```python
from build123d import *

# Parameters (mm, degrees)
F0_R     = 142.5
F1_DEPTH = 100
F2_R     = 100
F3_DEPTH = 75
F4_R     = 50
F5_DEPTH = 50


with BuildPart() as f1:
    # F0 (on Front) → F1 (new body)
    with BuildSketch(Plane.XZ):
        Circle(F0_R)
    extrude(amount=F1_DEPTH)

    # F2 (on face) → F3 (cut)
    with BuildSketch(Plane.XZ.offset(100)):
        Circle(F2_R)
    extrude(amount=-F3_DEPTH, mode=Mode.SUBTRACT)

    # F4 (on face) → F5 (join)
    with BuildSketch(Plane.XZ.offset(25)):
        Circle(F4_R)
    extrude(amount=F5_DEPTH)


solid = f1.part
```
For this review, take the finished solid that the model builds, in its own axes (mm). A direction names the side the tool comes from. Give positions to 0.01 mm unless a question says otherwise; leave off trailing zeros. Write each loop counter-clockwise with the first axis right and the second up, starting at its lowest first coordinate (ties: lowest second). Pieces come first, ordered by that corner, then holes. Notation, with made-up numbers: M 10.25,-13 L 53.25,-13 A26 ccw 53.25,15 Z; hole C 70,9.5 d3. An arc over 180 degrees is marked long. Answer as a JSON object with one key per item and string values. Group by question number.
Item 1: Consider section D-D on y = -86. Write out the cut boundary in (x, z), plus the area to 3 significant figures.
Item 2: For pin 1 Ø1.5 at (y, z) = (-85, -19.5) entering from +X; pin 2 Ø12 at (y, z) = (-79, -18) entering from +X; pin 3 Ø1 at (y, z) = (-19, -59.5) entering from +X, all flat-tipped, find the tip position at first contact; note any pin that passes through.
Item 3: For probe 1 along Z at (x, y) = (0, -73.5); probe 2 along Y at (x, z) = (67, 68); probe 3 along X at (y, z) = (-29.5, -51.5), list the stretches that pass through material, from the lowest coordinate up. Write a range as [from, to].
Item 4: Consider section C-C on z = 0. Write out the cut boundary in (x, y), plus the area to 3 significant figures.
Item 5: Consider section A-A on y = -70.5. Write out the cut boundary in (x, z), plus the area to 3 significant figures.
Item 6: Tool access review of faces 1 (the flat face through (-2, 0, 2)), 2 (the cylindrical face through (95.38, -63.02, 30.04)): name each direction out of +Z, -Z, +X, -X, +Y, -Y from which nothing blocks a thin tool from reaching the whole face with its end or side.
Item 7: Draft analysis for pull direction Z (two halves, no side actions). For faces 3 (the flat face through (30, -100, 97)), 4 (the cylindrical face through (-105.028, -49.3, 96.308)), 5 (the flat face through (-46, -25, -21)), state which applies: +Z half, -Z half, draft (parallel to the pull), parting line (faces both ways), or undercut.
Item 8: Consider section B-B on x = 0. Write out the cut boundary in (y, z).
Check result:
{
 "1": {"outline": "C 0,0 d285; hole C 0,0 d200", "area": "32,400 mm^2"},
 "2": {"pin 1": "stops at x = 141.26", "pin 2": "stops at x = 141.99", "pin 3": "stops at x = 129.71"},
 "3": {"probe 1": "z = [-142.5, -100], [-50, 50], [100, 142.5]", "probe 2": "y = [-25, 0]", "probe 3": "x = [-132.87, -85.72], [85.72, 132.87]"},
 "4": {"outline": "M -142.5,-100 L -100,-100 L -100,-25 L -50,-25 L -50,-75 L 50,-75 L 50,-25 L 100,-25 L 100,-100 L 142.5,-100 L 142.5,0 L -142.5,0 Z", "area": "18,500 mm^2"},
 "5": {"outline": "C 0,0 d285; C 0,0 d100; hole C 0,0 d200", "area": "40,200 mm^2"},
 "6": {"face 1": "+Z, -Z, +X, -X, +Y", "face 2": "-Y"},
 "7": {"face 3": "draft", "face 4": "parting line", "face 5": "undercut"},
 "8": {"outline": "M -100,-142.5 L 0,-142.5 L 0,142.5 L -100,142.5 L -100,100 L -25,100 L -25,50 L -75,50 L -75,-50 L -25,-50 L -25,-100 L -100,-100 Z"}
}
